Check sheet for the modelled part. Datum: model origin and axes. Units: mm. A direction names the side the tool comes from. Give positions to 0.01 mm unless a question says otherwise; leave off trailing zeros.
```python
from build123d import *

# Parameters (mm, degrees)
Y_KSEKLIK_EKSTR_ZYON1_DEPTH                    = 3
IZIM2_R                                        = 3.1
KES_EKSTR_ZYON1_DEPTH                          = 4
M2_D_Z_BA_L_MAKINE_VIDAS_IN_HAV_A1_D           = 2
M2_D_Z_BA_L_MAKINE_VIDAS_IN_HAV_A1_CSINK_D     = 2.6
M2_D_Z_BA_L_MAKINE_VIDAS_IN_HAV_A1_CSINK_ANGLE = 90
IZIM26_W                                       = 22.3
IZIM26_H                                       = 22
KES_EKSTR_ZYON4_DEPTH                          = 4
M2_D_Z_BA_L_MAKINE_VIDAS_IN_HAV_A2_D           = 2
M2_D_Z_BA_L_MAKINE_VIDAS_IN_HAV_A2_CSINK_D     = 2.6
M2_D_Z_BA_L_MAKINE_VIDAS_IN_HAV_A2_CSINK_ANGLE = 90
IZIM33_W                                       = 8
IZIM33_H                                       = 32
KES_EKSTR_ZYON5_DEPTH                          = 10
RADYUS1_R                                      = 0.5


with BuildPart() as part:
    # Çizim1 → Yükseklik-Ekstrüzyon1 (new body)
    with BuildSketch(Plane.XY):
        with BuildLine():
            ThreePointArc((-61, 16), (-77, 0), (-61, -16))
            Line((-61, -16), (75, -16))
            Line((75, -16), (75, 16))
            Line((75, 16), (-61, 16))
        make_face()
    extrude(amount=Y_KSEKLIK_EKSTR_ZYON1_DEPTH)

    # Çizim2 → Kes-Ekstrüzyon1 (cut, through all)
    with BuildSketch(Plane.XY.offset(3)):
        with Locations((-61, 0)):
            Circle(IZIM2_R)
    extrude(amount=-KES_EKSTR_ZYON1_DEPTH, mode=Mode.SUBTRACT)

    # M2 Düz Başlı Makine Vidası İçin Havşa1 (through all)
    with Locations(Plane(origin=(-61, 8, 3), x_dir=(1, 0, 0), z_dir=(0, 0, 1))):
        with Locations((0, 0), (8, -8), (0, -16), (-8, -8)):
            CounterSinkHole(M2_D_Z_BA_L_MAKINE_VIDAS_IN_HAV_A1_D / 2, M2_D_Z_BA_L_MAKINE_VIDAS_IN_HAV_A1_CSINK_D / 2, counter_sink_angle=M2_D_Z_BA_L_MAKINE_VIDAS_IN_HAV_A1_CSINK_ANGLE)

    # Çizim26 → Kes-Ekstrüzyon4 (cut, through all)
    with BuildSketch(Plane.XY.offset(3)):
        with Locations((63.85, 0)):
            Rectangle(IZIM26_W, IZIM26_H)
    extrude(amount=-KES_EKSTR_ZYON4_DEPTH, mode=Mode.SUBTRACT)

    # M2 Düz Başlı Makine Vidası İçin Havşa2 (through all)
    with Locations(Plane(origin=(71.7, 13.5, 0), x_dir=(-1, 0, 0), z_dir=(0, 0, -1))):
        with Locations((0, 0), (8, 0), (16, 0), (21.5, -5.5), (21.5, -21.5), (16, -27), (8, -27), (0, -27)):
            CounterSinkHole(M2_D_Z_BA_L_MAKINE_VIDAS_IN_HAV_A2_D / 2, M2_D_Z_BA_L_MAKINE_VIDAS_IN_HAV_A2_CSINK_D / 2, counter_sink_angle=M2_D_Z_BA_L_MAKINE_VIDAS_IN_HAV_A2_CSINK_ANGLE)

    # Çizim33 → Kes-Ekstrüzyon5 (cut)
    with BuildSketch(Plane(origin=(0, 0, 0), x_dir=(-1, 0, 0), z_dir=(0, 0, -1))):
        with Locations((-71, 0)):
            Rectangle(IZIM33_W, IZIM33_H)
    extrude(amount=-KES_EKSTR_ZYON5_DEPTH, mode=Mode.SUBTRACT)

    # Radyus1
    radyus1_edges = [part.edges().sort_by_distance(p)[0] for p in [
        (67, 11, 1.5),
        (67, -11, 1.5),
        (67, 16, 1.5),
        (67, -16, 1.5),
        (52.7, -11, 1.5),
        (52.7, 11, 1.5),
    ]]
    fillet(radyus1_edges, radius=RADYUS1_R)


solid = part.part
```
(1) Material ranges on L1, parallel to Y at x = 50.2, z = 1.45; L2, parallel to Y at x = -61, z = 2.25; L3, parallel to Y at x = 55.7, z = 1.65, recorded low to high.
Response values:
L1: y = -16 to -9, -7 to 7, 9 to 16
L2: y = -16 to -9, -7 to -3.1, 3.1 to 7, 9 to 16
L3: y = -16 to -14.5, -12.5 to -11, 11 to 12.5, 14.5 to 16
(2) Cross-section at A-A on z = 0.9. Count the separate pieces of the cut face and the enclosed holes in it, then the cut area to 3 significant figures.
Response values:
separate pieces: 1
enclosed holes: 11
area: 4,120 mm2
(3) Set-up check for faces 4 (the face through (-6, 0, 0)), 5 (the face through (60, -11, 2)): record each of +Z, -Z, +X, -X, +Y, -Y from which the full face is reachable in a straight line by a thin tool's end or side.
Response values:
face 4: -Z, +X, -X, +Y, -Y
face 5: +Z, -Z, +X
(4) Release check for a two-part mould opening along Y. For faces 1 (the face through (67, -14, 1)), 2 (the face through (52.7, 0, 2)), 3 (the face through (-77, 0, 1)) record: released by +Y, released by -Y, zero draft, split by the parting line, or undercut.
Response values:
face 1: zero draft
face 2: undercut
face 3: split by the parting line
(5) Gauge pin test, flat end, axial feed: pin 1 Ø2.5 at (x, y) = (63.7, 13.5) entering from -Z. Record the tip position at first contact, or that the pin passes through.
Response values:
pin 1: stops at z = 0.05
